Autodesk Inventor part; units mm, degrees
ref_plane "YZ Plane" through (0, 0, 0) normal (1, 0, 0) x (0, 1, 0)
ref_plane "XZ Plane" through (0, 0, 0) normal (0, 1, 0) x (-1, 0, 0)
ref_plane "XY Plane" through (0, 0, 0) normal (0, 0, 1) x (1, 0, 0)
sketch "Эскиз1" plane through (0, 0, 0) normal (0, 0, 1) x (1, 0, 0)
  line L0 (-13, 0) -> (13, 0)
  line L1 (-47.5, 180) -> (47.5, 180)
  line L2 (-16.5, 130) -> (16.5, 130)
  line L3 (-12.9827, 110) -> (12.9827, 110)
  line L4 (-11.8003, 90) -> (11.8003, 90)
  line L5 (47.5, 180) -> (37.594, 168.7363)
  line L6 (-47.5, 180) -> (-37.594, 168.7363)
  line L7 (-37.594, 168.7363) -> (37.594, 168.7363)
  arc A0 (37.594, 168.7363) -> (12.9827, 110) centre (112.573, 102.7948) ccw
  arc A1 (12.9827, 110) -> (13, 0) centre (771.5375, 55.1194) ccw
  arc A2 (-12.9827, 110) -> (-37.594, 168.7363) centre (-112.573, 102.7948) ccw
  arc A3 (-13, 0) -> (-12.9827, 110) centre (-771.5375, 55.1194) ccw
  line L8 (-11, 80.4723) -> (-11, 26.1046)
  line L9 (11, 80.4723) -> (11, 26.1046)
  line L10 (-37.594, 168.7363) -> (13.0707, 111.1279)
  line L11 (37.594, 168.7363) -> (-13.0707, 111.1279)
  point P0 (0, 0)
  point P1 (0, 0)
  point P2 (0, 180)
  point P3 (0, 130)
  point P4 (0, 90)
  point P5 (0, 110)
  point P6 (-11, 55.1194)
  dimension "d0" = 26
  dimension "d1" = 95
  dimension "d2" = 33
  dimension "d5" = 180
  dimension "d6" = 50
  dimension "d7" = 20
  dimension "d8" = 20
  dimension "d9" = 15
  dimension "d10" = 15
  dimension "d13" = 22
  dimension "d19" = 55.1194
extrude "Выдавливание1" add sketch "Эскиз1" along normal blind 25
sketch "Эскиз2" plane through (0, 0, 0) normal (1, 0, 0) x (0, 1, 0)
  line L0 (0, 0) -> (110, 0)
  line L1 (110, 0) -> (110, 25)
  line L2 (0, 25) -> (110, 25)
  line L3 (0, 0) -> (0, 25)
  line L4 (110, 0) -> (169.3956, 0)
  line L5 (110, 25) -> (169.3956, 25)
  line L6 (110, 0) -> (110, 25)
  line L7 (130, 18) -> (130, 7)
  line L8 (55, 21) -> (55, 4)
  arc A0 (0, 25) -> (130, 18) centre (172.2556, 2013.3889) ccw
  arc A1 (130, 7) -> (0, 0) centre (172.2556, -1988.3889) ccw
  line L9 (180, 13) -> (180, 12)
  line L10 (160, 14.5) -> (160, 10.5)
  line L11 (180, 13) -> (160, 14.5)
  line L12 (180, 12) -> (160, 10.5)
  arc A2 (130, 18) -> (160, 14.5) centre (187.3675, 379.4) ccw
  arc A3 (160, 10.5) -> (130, 7) centre (187.3675, -354.4) ccw
  line L13 (168.7363, 0) -> (180, 0)
  line L14 (180, 0) -> (180, 25)
  line L15 (168.7363, 25) -> (180, 25)
  line L16 (160, 13.75) -> (156, 13.75)
  line L17 (156, 13.75) -> (156, 11.25)
  line L18 (156, 11.25) -> (160, 11.25)
  point P0 (130, 12.5)
  point P1 (0, 12.5)
  point P2 (55, 12.5)
  point P3 (180, 12.5)
  point P4 (169.3956, 12.5)
  point P5 (160, 12.5)
  point P6 (180, 12.5)
  point P7 (156, 12.5)
  dimension "d16" = 11
  dimension "d20" = 55
  dimension "d21" = 17
  dimension "d22" = 1
  dimension "d23" = 4
  dimension "d28" = 50
  dimension "d30" = 20
  dimension "d33" = 4
  dimension "d34" = 2.5
extrude "Выдавливание2" cut sketch "Эскиз2" along normal mid plane 100 contours L10 L11 L9 L12 | L18 L17 L16 L10 keep common part
properties part number "bachi_v2" material "Фарфор, слоновая кость"
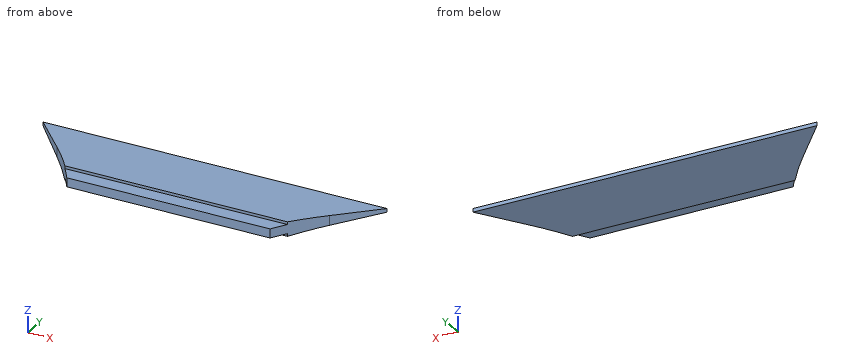
Geometry check sheet. Reference: the model listing, model coordinates, mm. Coordinates: 2 decimals unless noted, no trailing zeros. Order: outer loops, then holes, each group sorted by start corner. A loop starts at its lowest first (then second) coordinate and runs counter-clockwise, first axis right, second up. Notation, with made-up numbers: (-15.5, 66) - (2.5, 66) arc R6 ccw to (2.5, 70) - close; hole circle Ø4 at (4, 88). An arc over 180 degrees is marked (long way). Answer as a JSON object with one key per item and string values. Group by question number.
Item 1: Sectioned sample at B-B, the plane y = 170.25. Record the cut outline in (x, z), and give its area (3 significant figures).
Item 2: Sectioned sample at A-A, the plane x = 23. Record the cut outline in (y, z).
Item 3: Sectioned sample at C-C, the plane y = 162.25. Record the cut outline in (x, z), and give its area (3 significant figures).
Item 4: Scan lines: probe 1 along Z at (x, y) = (-28.5, 169.75); probe 2 along Z at (x, y) = (-25.5, 170); probe 3 along Y at (x, z) = (30.5, 12.05). Record each from-to range of solid material in increasing order.
Item 5: Depth check by flat-ended pin: pin 1 Ø1 at (y, z) = (170, 11.5) entering from +X; pin 2 Ø5 at (x, y) = (-31.5, 168) entering from +Z; pin 3 Ø2 at (y, z) = (164.5, 11) entering from -X; pin 4 Ø4.5 at (x, y) = (-2, 158.5) entering from -Z. Enter the tip coordinate at first touch or a pass-through.
Resolved:
{
 "1": {"outline": "(-38.93, 11.27) - (38.93, 11.27) - (38.93, 13.73) - (-38.93, 13.73) - close", "area": "192 mm^2"},
 "2": {"outline": "(156, 11.25) - (160, 11.25) - (160, 10.5) - (180, 12) - (180, 13) - (160, 14.5) - (160, 13.75) - (156, 13.75) - close"},
 "3": {"outline": "(-32.35, 10.67) - (32.35, 10.67) - (32.35, 14.33) - (-32.35, 14.33) - close", "area": "237 mm^2"},
 "4": {"probe 1": "11.23 to 13.77", "probe 2": "11.25 to 13.75", "probe 3": "159.66 to 180"},
 "5": {"pin 1": "x = 39.15", "pin 2": "z = 14.09", "pin 3": "x = -34.87", "pin 4": "z = 10.5"}
}
